Check sheet for the modelled part. Datum: model origin and axes. Units: mm. A direction names the side the tool comes from. Give positions to 0.01 mm unless a question says otherwise; leave off trailing zeros. Write each loop counter-clockwise with the first axis right and the second up, starting at its lowest first coordinate (ties: lowest second). Pieces come first, ordered by that corner, then holes. Notation, with made-up numbers: M 22.5,39 L 69.5,39 A25 cw 69.5,74 Z; hole C 49.25,-31.5 d4. An arc over 180 degrees is marked long. Write item = value, one per line. Start each with the question number.
1) Access from +Z, -Z, +X, -X, +Y, -Y to the whole of each face (thin tool, end or side, straight path). Record for faces 1 (the cylindrical face through (25.425, 4.493, 45.786)), 2 (the flat face through (14, 1, 25)).
2) Scan lines: line 1 along Z through (x, y) = (2.75, 4.3); line 2 along X through (y, z) = (0.6, 47.25); line 3 along Y through (x, z) = (15.25, 4.5). Record each from-to range of solid material in increasing order. Write a range as [from, to].
3) Mould release check, pull along X, two halves, no side actions. Record for faces 3 (the cylindrical face through (2.425, 0.493, 1.286)), 4 (the flat face through (14.1, 0.8, 0)), 5 (the flat face through (28.5, 2, 25)): released by +X, released by -X, zero draft, split by the parting line, or undercut.
4) Go/stop test with a flat-tipped pin: pin 1 (1.5 mm diameter, centred on x = 16, y = 4, fed in from -Z). Record where the tip stops, or that it passes through.
5) Cross-section at A-A, the plane x = 12.5. Record the cut outline in (y, z), plus the area to 3 significant figures.
6) Cross-section at B-B, the plane z = 2.75. Record the cut outline in (x, y), plus the area to 3 significant figures.
7) Cross-section at D-D, the plane x = 2.75. Record the cut outline in (y, z), plus the area to 3 significant figures.
8) Cross-section at C-C, the plane y = 1.8. Record the cut outline in (x, z).
Autodesk Fusion 360 part; units mm, degrees
sketch "Esquisse1" plane through (0, 0, 0) normal (0, 1, 0) x (1, 0, 0)
  line L0 (0, 0) -> (28.5, 0)
  line L1 (28.5, 0) -> (28.5, -50)
  line L2 (28.5, -50) -> (0, -50)
  line L3 (0, -50) -> (0, 0)
  circle A0 centre (2.75, -2.75) radius 1.5
  circle A1 centre (25.75, -2.75) radius 1.5
  circle A2 centre (2.75, -47.25) radius 1.5
  circle A3 centre (25.75, -47.25) radius 1.5
  dimension "d1" = 28.5
  dimension "d2" = 50
  dimension "d3" = 3
  dimension "d4" = 3
  dimension "d5" = 3
  dimension "d6" = 3
  dimension "d7" = 2.75
  dimension "d8" = 2.75
  dimension "d9" = 2.75
  dimension "d10" = 2.75
  dimension "d11" = 2.75
  dimension "d12" = 2.75
  dimension "d13" = 2.75
  dimension "d14" = 2.75
extrude "Extrusion1" add sketch "Esquisse1" along normal blind 5
sketch "Esquisse2" plane through (0, 0, 0) normal (0, 0, -1) x (-1, 0, 0)
  line L0 (-28.5, 0) -> (0, 0)
  line L1 (0, 0) -> (0, 5)
  line L2 (0, 5) -> (-28.5, 5)
  line L3 (-28.5, 5) -> (-28.5, 0)
  line L4 (-27.5, 4) -> (-1, 4)
  line L5 (-1, 4) -> (-1, 1)
  line L6 (-1, 1) -> (-27.5, 1)
  line L7 (-27.5, 1) -> (-27.5, 4)
  dimension "d17" = 1
  dimension "d18" = 1
  dimension "d19" = 1
  dimension "d20" = 1
extrude "Extrusion2" cut sketch "Esquisse2" against normal blind 71 contours L4 L5 L6 L7
sketch "Esquisse3" plane through (0, 5, 0) normal (0, 1, 0) x (-1, 0, 0)
  circle A0 centre (-2.75, 2.75) radius 1.5
  circle A1 centre (-2.75, 47.25) radius 1.5
  circle A2 centre (-25.75, 2.75) radius 1.5
  circle A3 centre (-25.75, 47.25) radius 1.5
  line L0 (0, 50) -> (-28.5, 50)
  line L1 (-28.5, 50) -> (-28.5, 0)
  line L2 (-28.5, 0) -> (0, 0)
  line L3 (0, 0) -> (0, 50)
Reply:
q1.face_1 = +Y, -Y
q1.face_2 = +Z, -Z
q2.line_1 = [0, 1.25], [4.25, 45.75], [48.75, 50]
q2.line_2 = [0, 1.25], [4.25, 24.25], [27.25, 28.5]
q2.line_3 = [0, 1], [4, 5]
q3.face_3 = undercut
q3.face_4 = zero draft
q3.face_5 = released by +X
q4.pin_1 = 0
q5.outline = M 0,0 L 1,0 L 1,50 L 0,50 Z; M 4,0 L 5,0 L 5,50 L 4,50 Z
q5.area = 100 mm2
q6.outline = M 0,0 L 1.25,0 L 1.25,1 L 1,1 L 1,4 L 1.25,4 L 1.25,5 L 0,5 Z; M 4.25,0 L 24.25,0 L 24.25,1 L 4.25,1 Z; M 4.25,4 L 24.25,4 L 24.25,5 L 4.25,5 Z; M 27.25,0 L 28.5,0 L 28.5,5 L 27.25,5 L 27.25,4 L 27.5,4 L 27.5,1 L 27.25,1 Z
q6.area = 51.0 mm2
q7.outline = M 0,0 L 1,0 L 1,1.25 L 0,1.25 Z; M 0,4.25 L 1,4.25 L 1,45.75 L 0,45.75 Z; M 0,48.75 L 1,48.75 L 1,50 L 0,50 Z; M 4,0 L 5,0 L 5,1.25 L 4,1.25 Z; M 4,4.25 L 5,4.25 L 5,45.75 L 4,45.75 Z; M 4,48.75 L 5,48.75 L 5,50 L 4,50 Z
q7.area = 88.0 mm2
q8.outline = M 0,0 L 1,0 L 1,50 L 0,50 Z; M 27.5,0 L 28.5,0 L 28.5,50 L 27.5,50 Z
